from build123d import *

# Parameters (mm, degrees)
SKETCH1_R           = 6.096
BOSS_EXTRUDE1_DEPTH = 9.525
SKETCH2_R           = 2.5527
CUT_EXTRUDE1_DEPTH  = 4.175
SKETCH3_R           = 9.271
SKETCH3_R_2         = 6.096
BOSS_EXTRUDE2_DEPTH = 2.794
SKETCH6_R           = 9.906
SKETCH6_R_2         = 8.636
BOSS_EXTRUDE4_DEPTH = 12.319
SKETCH5_R           = 8.636
CUT_EXTRUDE2_DEPTH  = 12.319
SKETCH4_R           = 9.906
SKETCH4_R_2         = 7.366
BOSS_EXTRUDE3_DEPTH = 1.27


with BuildPart() as part:
    # Sketch1 → Boss-Extrude1 (new body)
    with BuildSketch(Plane(origin=(0, 0, 0), x_dir=(1, 0, 0), z_dir=(0, 1, 0))):
        with BuildLine():
            Line((-9.271, 0), (-9.271, 10.668))
            Line((-9.271, 10.668), (-18.796, 10.668))
            Line((-18.796, 10.668), (-18.796, 13.843))
            Line((-18.796, 13.843), (-6.096, 13.843))
            Line((-6.096, 13.843), (6.096, 13.843))
            Line((6.096, 13.843), (18.796, 13.843))
            Line((18.796, 13.843), (18.796, 10.668))
            Line((18.796, 10.668), (9.271, 10.668))
            Line((9.271, 10.668), (9.271, 0))
            ThreePointArc((9.271, 0), (0, -9.271), (-9.271, 0))
        make_face()
        Circle(SKETCH1_R, mode=Mode.SUBTRACT)
        with BuildLine():
            Line((-6.096, 6.731), (-6.096, 10.668))
            Line((-6.096, 10.668), (6.096, 10.668))
            Line((6.096, 10.668), (6.096, 6.731))
            ThreePointArc((6.096, 6.731), (0, 9.081166059), (-6.096, 6.731))
        make_face(mode=Mode.SUBTRACT)
    extrude(amount=BOSS_EXTRUDE1_DEPTH)

    # Sketch2 → Cut-Extrude1 (cut, through all)
    with BuildSketch(Plane.XY.offset(-10.668)):
        with Locations((-14.0335, 4.7625)):
            Circle(SKETCH2_R)
        with Locations((14.0335, 4.7625)):
            Circle(SKETCH2_R)
    extrude(amount=-CUT_EXTRUDE1_DEPTH, mode=Mode.SUBTRACT)

    # Sketch3 → Boss-Extrude2 (add)
    with BuildSketch(Plane(origin=(0, 0, 0), x_dir=(-1, 0, 0), z_dir=(0, -1, 0))):
        Circle(SKETCH3_R)
        Circle(SKETCH3_R_2, mode=Mode.SUBTRACT)
    extrude(amount=BOSS_EXTRUDE2_DEPTH)

    # Sketch6 → Boss-Extrude4 (add)
    with BuildSketch(Plane(origin=(0, 9.525, 0), x_dir=(1, 0, 0), z_dir=(0, 1, 0))):
        Circle(SKETCH6_R)
        Circle(SKETCH6_R_2, mode=Mode.SUBTRACT)
    extrude(amount=-BOSS_EXTRUDE4_DEPTH)

    # Sketch5 → Cut-Extrude2 (cut)
    with BuildSketch(Plane(origin=(0, 9.525, 0), x_dir=(1, 0, 0), z_dir=(0, 1, 0))):
        Circle(SKETCH5_R)
    extrude(amount=-CUT_EXTRUDE2_DEPTH, mode=Mode.SUBTRACT)

    # Sketch4 → Boss-Extrude3 (add)
    with BuildSketch(Plane(origin=(0, -2.794, 0), x_dir=(-1, 0, 0), z_dir=(0, -1, 0))):
        Circle(SKETCH4_R)
        Circle(SKETCH4_R_2, mode=Mode.SUBTRACT)
    extrude(amount=BOSS_EXTRUDE3_DEPTH)


solid = part.part
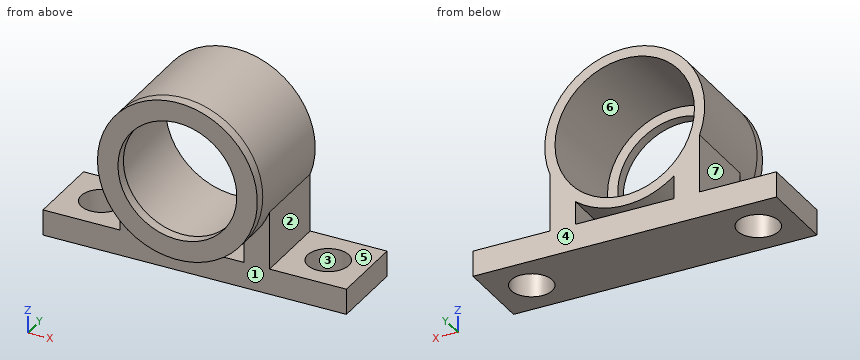
Work out the finished part from the listing and answer in its coordinate system (mm). Face numbers are marked on the shaded views. A direction names the side the tool comes from. Coordinates: 2 decimals unless noted, no trailing zeros. Order: outer loops, then holes, each group sorted by start corner. A loop starts at its lowest first (then second) coordinate and runs counter-clockwise, first axis right, second up. Notation, with made-up numbers: (-33, 88.5) - (-21, 88.5) arc R29 ccw to (-21, 127.5) - close; hole circle Ø10 at (-11, -3.75). An arc over 180 degrees is marked (long way). Put each result on its own line as item: value. Start each with the question number.
1) For the marked faces 4, 5, 6 and 7, determine the directions among +Z, -Z, +X, -X, +Y, -Y from which every point of the face is accessible in a straight line to the end or side of a thin tool.
2) Find the intervals of material crossed by line 1 (Z direction, x = 0, y = 6); line 2 (X direction, y = -3.6, z = 0); line 3 (Z direction, x = 1.5, y = 8.25), in increasing order. Write a range as from..to.
3) For a pull along Y with two mould halves and no side action, classify the marked faces 1, 2 and 3 as released by +Y, released by -Y, zero draft, split by the parting line, or undercut.
4) Find section D-D (y = -0.5). Give the vertices of the cut face in (x, z), plus the area to 3 significant figures.
5) Flat-ended cylindrical pins translate along their axes: pin 1 (1.4 mm diameter, centred on y = 3, z = -9.5, fed in from +X); pin 2 (0.9 mm diameter, centred on y = 5, z = -8.5, fed in from -X); pin 3 (3 mm diameter, centred on y = 2.5, z = -9.5, fed in from +X); pin 4 (3 mm diameter, centred on x = 15, y = 3, fed in from +Z). Find the tip coordinate at first contact, or state that the pin passes through.
6) Find section B-B (z = 0). Give the vertices of the cut face in (x, y) (3 decimals).
7) Find section A-A (x = 0). Give the vertices of the cut face in (y, z) (3 decimals).
8) Find section C-C (y = 8.5). Give the vertices of the cut face in (x, z).
Results list:
1. face 4: +Z, -Z, +X, -X, +Y
1. face 5: +X, +Y, -Y
1. face 6: +Y
1. face 7: -X, +Y, -Y
2. line 1: z = -13.84..-10.67, -9.91..-8.64, 8.64..9.91
2. line 2: x = -9.91..-7.37, 7.37..9.91
2. line 3: z = -13.84..-10.67, -9.79..-8.5, 8.5..9.79
3. face 1: released by -Y
3. face 2: zero draft
3. face 3: undercut
4. outline: circle Ø19.81 at (0, 0); hole circle Ø17.27 at (0, 0)
4. area: 74.0 mm^2
5. pin 1: stops at x = 9.27
5. pin 2: stops at x = -9.27
5. pin 3: stops at x = 18.8
5. pin 4: stops at z = -10.67
6. outline: (-9.906, -4.064) - (-7.366, -4.064) - (-7.366, -2.794) - (-8.636, -2.794) - (-8.636, 9.525) - (-9.906, 9.525) - close; (7.366, -4.064) - (9.906, -4.064) - (9.906, 9.525) - (8.636, 9.525) - (8.636, -2.794) - (7.366, -2.794) - close
7. outline: (-4.064, -9.906) - (9.525, -9.906) - (9.525, -8.636) - (-2.794, -8.636) - (-2.794, -7.366) - (-4.064, -7.366) - close; (-4.064, 7.366) - (-2.794, 7.366) - (-2.794, 8.636) - (9.525, 8.636) - (9.525, 9.906) - (-4.064, 9.906) - close; (0, -13.843) - (9.525, -13.843) - (9.525, -10.668) - (0, -10.668) - close
8. outline: (-18.8, -13.84) - (18.8, -13.84) - (18.8, -10.67) - (9.27, -10.67) - (9.27, -3.49) arc R9.91 ccw (long way) to (-9.27, -3.49) - (-9.27, -10.67) - (-18.8, -10.67) - close; hole circle Ø17.27 at (0, 0); hole (-6.1, -10.67) - (6.1, -10.67) - (6.1, -7.81) arc R9.91 cw to (-6.1, -7.81) - close
